Input: part model. Units: mm. Frame: model coordinates. A direction names the side the tool comes from. Give positions to 0.01 mm unless a question says otherwise; leave off trailing zeros. Loops run counter-clockwise (first coordinate to the right, second up) from the corner with the lowest first, then second, coordinate; pieces in that order, holes last. Notation, with made-up numbers: (27, 54.5) - (36, 54.5) arc R19 ccw to (36, 59.5) - close; hole circle Ø10 at (-18, 57). An arc over 180 degrees is marked (long way). Answer as a JSON object with one key per item and string values. Group by question number.
(1) Material intervals for L1, parallel to Y at x = 46, z = 3.5; L2, parallel to Z at x = -50.5, y = 17.25; L3, parallel to Z at x = 42.5, y = 9.75, sorted ascending.
(2) Section query B-B (x = -17). Return loops of the section in (y, z) (3 decimals), plus the area to 3 significant figures.
(3) Mould query, pull axis X, two halves, no side actions, for faces 1 (the cylindrical face through (-0.867, 10.383, -16.587)), 2 (the cylindrical face through (48.4, 25.15, -16.61)), 3 (the flat face through (-1, 0, 0)). Classes: +X half, -X half, draft (parallel to the pull), parting line (faces both ways), or undercut.
(4) Section query A-A (x = 0). Return loops of the section in (y, z), plus the area to 4 significant figures.
(5) Section query C-C (x = 25). Return loops of the section in (y, z), plus the area to 3 significant figures.
(6) Access query for faces 4 (the cylindrical face through (11.195, 0.751, 16.759)), 5 (the cylindrical face through (-55.207, 0.773, -4.883)). Directions: +Z, -Z, +X, -X, +Y, -Y. A direction counts if a zero-diameter tool reaches every point of the face in a straight line with its end or side. Return the directions, or none.
(7) Pin query (flat end, axial travel): P1, Ø1.3, axis at x = -11.41, z = 5.36, coming from the -Y side; P2, Ø3, axis at y = 2.5, z = -1.5, coming from the -X side; P3, Ø0.5, axis at x = 9.5, y = 1, coming from the +Z side; P4, Ø7, axis at x = -53.075, z = 5.5, coming from the +Y side. Return the tip coordinate at first contact, or that it passes through.
```python
from build123d import *

# Parameters (mm, degrees)
SKETCH1_W               = 114.3
SKETCH1_H               = 34.72
BOSS_EXTRUDE1_DEPTH     = 1.524
SKETCH2_R               = 2.184
SKETCH2_W               = 8.15
SKETCH2_H               = 6.35
CUT_EXTRUDE1_DEPTH      = 1.524
SKETCH3_R               = 4
CUT_EXTRUDE2_DEPTH      = 50
SKETCH4_R               = 1.09
CUT_EXTRUDE3_DEPTH      = 50
CIRPATTERN1_COUNT       = 4
MIRROR2_COPY_1_SKETCH_R = 1.09
MIRROR2_COPY_1_DEPTH    = 50
MIRROR2_COPY_2_SKETCH_R = 1.09
MIRROR2_COPY_2_DEPTH    = 50
MIRROR2_COPY_3_SKETCH_R = 1.09
MIRROR2_COPY_3_DEPTH    = 50
SKETCH7_R               = 4
CUT_EXTRUDE4_DEPTH      = 100
SKETCH8_R               = 1.09
CUT_EXTRUDE5_DEPTH      = 100
CIRPATTERN2_COUNT       = 4
MIRROR3_COPY_1_SKETCH_R = 1.09
MIRROR3_COPY_1_DEPTH    = 50
MIRROR3_COPY_2_SKETCH_R = 1.09
MIRROR3_COPY_2_DEPTH    = 50
MIRROR3_COPY_3_SKETCH_R = 1.09
MIRROR3_COPY_3_DEPTH    = 50
MIRROR3_COPY_4_SKETCH_R = 4
MIRROR3_COPY_4_DEPTH    = 50
MIRROR3_COPY_5_SKETCH_R = 1.09
MIRROR3_COPY_5_DEPTH    = 50
MIRROR3_COPY_6_SKETCH_R = 1.09
MIRROR3_COPY_6_DEPTH    = 50
MIRROR3_COPY_7_SKETCH_R = 1.09
MIRROR3_COPY_7_DEPTH    = 50
MIRROR3_COPY_8_SKETCH_R = 1.09
MIRROR3_COPY_8_DEPTH    = 50
SKETCH9_W               = 7.9375
SKETCH9_H               = 1.524
BOSS_EXTRUDE2_DEPTH     = 24.2
SKETCH10_W              = 98
SKETCH10_H              = 1.524
SKETCH10_W_2            = 18.075
BOSS_EXTRUDE3_DEPTH     = 24.2
SKETCH11_R              = 2.1844
CUT_EXTRUDE6_DEPTH      = 24.2
SKETCH12_R              = 2.1844
CUT_EXTRUDE8_DEPTH      = 24.2
FILLET1_R               = 1
SKETCH13_R              = 1.5875
CUT_EXTRUDE9_DEPTH      = 24.2
FILLET2_R               = 2
SKETCH14_R              = 4
CUT_EXTRUDE10_DEPTH     = 24.2
SKETCH15_R              = 1.09
CUT_EXTRUDE11_DEPTH     = 24.2
CIRPATTERN3_COUNT       = 4


with BuildPart() as part:
    # Sketch1 → Boss-Extrude1 (new body)
    with BuildSketch(Plane(origin=(0, 0, 0), x_dir=(1, 0, 0), z_dir=(0, 1, 0))):
        Rectangle(SKETCH1_W, SKETCH1_H)
    extrude(amount=BOSS_EXTRUDE1_DEPTH)

    # Sketch2 → Cut-Extrude1 (cut)
    with BuildSketch(Plane(origin=(0, 1.524, 0), x_dir=(1, 0, 0), z_dir=(0, 1, 0))):
        with Locations(Location((-53.075, 4.41, 0), (0, 0, 270))):
            Circle(SKETCH2_R)
        with Locations(Location((-53.075, -5.5, 0), (0, 0, 270))):
            Circle(SKETCH2_R)
        with Locations((-53.075, 14.185)):
            Rectangle(SKETCH2_W, SKETCH2_H)
        Polygon((-57.15, -13.36), (-49.2125, -13.36), (-49.2125, -9.16), (-47.625, -9.16), (-47.625, -13.36), (-47.625, -17.36), (-57.15, -17.36), align=None)
        Polygon((-10.625, -13.36), (-10.625, -9.16), (-9.0375, -9.16), (-9.0375, -13.36), (0, -13.36), (0, -17.36), (-10.625, -17.36), align=None)
    cut_extrude1 = extrude(amount=-CUT_EXTRUDE1_DEPTH, mode=Mode.SUBTRACT)

    # Mirror1: Cut-Extrude1 across plane
    add(cut_extrude1.mirror(Plane(origin=(0, 0, 0), x_dir=(0, 0, 1), z_dir=(1, 0, 0))), mode=Mode.SUBTRACT)

    # Sketch3 → Cut-Extrude2 (cut, symmetric)
    with BuildSketch(Plane(origin=(0, 1.524, 0), x_dir=(1, 0, 0), z_dir=(0, 1, 0))):
        with Locations(Location((-36.9062, -5.36, 0), (0, 0, 90))):
            Circle(SKETCH3_R)
    cut_extrude2 = extrude(amount=CUT_EXTRUDE2_DEPTH, both=True, mode=Mode.SUBTRACT)

    # Sketch4 → Cut-Extrude3 (cut, symmetric)
    with BuildSketch(Plane(origin=(0, 1.524, 0), x_dir=(1, 0, 0), z_dir=(0, 1, 0))):
        with Locations(Location((-36.9062, 3.14, 0), (0, 0, 90))):
            Circle(SKETCH4_R)
    cut_extrude3 = extrude(amount=CUT_EXTRUDE3_DEPTH, both=True, mode=Mode.SUBTRACT)

    # CirPattern1: Cut-Extrude3 ×4 about axis
    cirpattern1_axis = Axis((-36.9062, 0, 5.36), (0, 1, 0))
    for i in range(1, CIRPATTERN1_COUNT):
        add(cut_extrude3.rotate(cirpattern1_axis, i * 360 / CIRPATTERN1_COUNT), mode=Mode.SUBTRACT)

    # Mirror2: Cut-Extrude2, Cut-Extrude3 across plane
    add(cut_extrude2.mirror(Plane.ZY.offset(28.4062)), mode=Mode.SUBTRACT)
    add(cut_extrude3.mirror(Plane.ZY.offset(28.4062)), mode=Mode.SUBTRACT)

    # Mirror2 copy 1 sketch → Mirror2 copy 1 (cut, symmetric)
    with BuildSketch(Plane(origin=(-14.5462, 1.524, -31.5462), x_dir=(0, 0, -1), z_dir=(0, 1, 0))):
        with Locations((-36.9062, -3.14)):
            Circle(MIRROR2_COPY_1_SKETCH_R)
    extrude(amount=MIRROR2_COPY_1_DEPTH, both=True, mode=Mode.SUBTRACT)

    # Mirror2 copy 2 sketch → Mirror2 copy 2 (cut, symmetric)
    with BuildSketch(Plane(origin=(17, 1.524, 10.72), x_dir=(1, 0, 0), z_dir=(0, 1, 0))):
        with Locations((-36.9062, -3.14)):
            Circle(MIRROR2_COPY_2_SKETCH_R)
    extrude(amount=MIRROR2_COPY_2_DEPTH, both=True, mode=Mode.SUBTRACT)

    # Mirror2 copy 3 sketch → Mirror2 copy 3 (cut, symmetric)
    with BuildSketch(Plane(origin=(-25.2662, 1.524, 42.2662), x_dir=(0, 0, 1), z_dir=(0, 1, 0))):
        with Locations((-36.9062, -3.14)):
            Circle(MIRROR2_COPY_3_SKETCH_R)
    extrude(amount=MIRROR2_COPY_3_DEPTH, both=True, mode=Mode.SUBTRACT)

    # Sketch7 → Cut-Extrude4 (cut)
    with BuildSketch(Plane(origin=(0, 1.524, 0), x_dir=(1, 0, 0), z_dir=(0, 1, 0))):
        with Locations(Location((0, -5.36, 0), (0, 0, 270))):
            Circle(SKETCH7_R)
    extrude(amount=-CUT_EXTRUDE4_DEPTH, mode=Mode.SUBTRACT)

    # Sketch8 → Cut-Extrude5 (cut)
    with BuildSketch(Plane(origin=(0, 1.524, 0), x_dir=(1, 0, 0), z_dir=(0, 1, 0))):
        with Locations(Location((0, 3.14, 0), (0, 0, 270))):
            Circle(SKETCH8_R)
    cut_extrude5 = extrude(amount=-CUT_EXTRUDE5_DEPTH, mode=Mode.SUBTRACT)

    # CirPattern2: Cut-Extrude5 ×4 about axis, 1 skipped
    cirpattern2_axis = Axis((0, 0, 5.36), (0, 1, 0))
    add([cut_extrude5.rotate(cirpattern2_axis, i * 360 / CIRPATTERN2_COUNT) for i in range(1, CIRPATTERN2_COUNT) if i not in (2,)], mode=Mode.SUBTRACT)

    # Mirror3: Cut-Extrude2, Cut-Extrude3 across plane
    add(cut_extrude2.mirror(Plane(origin=(0, 0, 0), x_dir=(0, 0, 1), z_dir=(1, 0, 0))), mode=Mode.SUBTRACT)
    add(cut_extrude3.mirror(Plane(origin=(0, 0, 0), x_dir=(0, 0, 1), z_dir=(1, 0, 0))), mode=Mode.SUBTRACT)

    # Mirror3 copy 1 sketch → Mirror3 copy 1 (cut, symmetric)
    with BuildSketch(Plane(origin=(42.2662, 1.524, -31.5462), x_dir=(0, 0, -1), z_dir=(0, 1, 0))):
        with Locations((-36.9062, -3.14)):
            Circle(MIRROR3_COPY_1_SKETCH_R)
    extrude(amount=MIRROR3_COPY_1_DEPTH, both=True, mode=Mode.SUBTRACT)

    # Mirror3 copy 2 sketch → Mirror3 copy 2 (cut, symmetric)
    with BuildSketch(Plane(origin=(73.8124, 1.524, 10.72), x_dir=(1, 0, 0), z_dir=(0, 1, 0))):
        with Locations((-36.9062, -3.14)):
            Circle(MIRROR3_COPY_2_SKETCH_R)
    extrude(amount=MIRROR3_COPY_2_DEPTH, both=True, mode=Mode.SUBTRACT)

    # Mirror3 copy 3 sketch → Mirror3 copy 3 (cut, symmetric)
    with BuildSketch(Plane(origin=(31.5462, 1.524, 42.2662), x_dir=(0, 0, 1), z_dir=(0, 1, 0))):
        with Locations((-36.9062, -3.14)):
            Circle(MIRROR3_COPY_3_SKETCH_R)
    extrude(amount=MIRROR3_COPY_3_DEPTH, both=True, mode=Mode.SUBTRACT)

    # Mirror3 copy 4 sketch → Mirror3 copy 4 (cut, symmetric)
    with BuildSketch(Plane(origin=(56.8124, 1.524, 0), x_dir=(1, 0, 0), z_dir=(0, 1, 0))):
        with Locations(Location((-36.9062, -5.36, 0), (0, 0, 90))):
            Circle(MIRROR3_COPY_4_SKETCH_R)
    extrude(amount=MIRROR3_COPY_4_DEPTH, both=True, mode=Mode.SUBTRACT)

    # Mirror3 copy 5 sketch → Mirror3 copy 5 (cut, symmetric)
    with BuildSketch(Plane(origin=(56.8124, 1.524, 0), x_dir=(1, 0, 0), z_dir=(0, 1, 0))):
        with Locations(Location((-36.9062, 3.14, 0), (0, 0, 90))):
            Circle(MIRROR3_COPY_5_SKETCH_R)
    extrude(amount=MIRROR3_COPY_5_DEPTH, both=True, mode=Mode.SUBTRACT)

    # Mirror3 copy 6 sketch → Mirror3 copy 6 (cut, symmetric)
    with BuildSketch(Plane(origin=(14.5462, 1.524, -31.5462), x_dir=(0, 0, -1), z_dir=(0, 1, 0))):
        with Locations(Location((-36.9062, 3.14, 0), (0, 0, 90))):
            Circle(MIRROR3_COPY_6_SKETCH_R)
    extrude(amount=MIRROR3_COPY_6_DEPTH, both=True, mode=Mode.SUBTRACT)

    # Mirror3 copy 7 sketch → Mirror3 copy 7 (cut, symmetric)
    with BuildSketch(Plane(origin=(-17, 1.524, 10.72), x_dir=(-1, 0, 0), z_dir=(0, 1, 0))):
        with Locations(Location((-36.9062, 3.14, 0), (0, 0, 90))):
            Circle(MIRROR3_COPY_7_SKETCH_R)
    extrude(amount=MIRROR3_COPY_7_DEPTH, both=True, mode=Mode.SUBTRACT)

    # Mirror3 copy 8 sketch → Mirror3 copy 8 (cut, symmetric)
    with BuildSketch(Plane(origin=(25.2662, 1.524, 42.2662), x_dir=(0, 0, 1), z_dir=(0, 1, 0))):
        with Locations(Location((-36.9062, 3.14, 0), (0, 0, 90))):
            Circle(MIRROR3_COPY_8_SKETCH_R)
    extrude(amount=MIRROR3_COPY_8_DEPTH, both=True, mode=Mode.SUBTRACT)

    # Sketch9 → Boss-Extrude2 (add)
    with BuildSketch(Plane(origin=(0, 1.524, 0), x_dir=(1, 0, 0), z_dir=(0, 1, 0))):
        with Locations((-53.18125, -12.598)):
            Rectangle(SKETCH9_W, SKETCH9_H)
    boss_extrude2 = extrude(amount=BOSS_EXTRUDE2_DEPTH)

    # Mirror4: Boss-Extrude2 across plane
    add(boss_extrude2.mirror(Plane(origin=(0, 0, 0), x_dir=(0, 0, 1), z_dir=(1, 0, 0))))

    # Sketch10 → Boss-Extrude3 (add)
    with BuildSketch(Plane(origin=(0, 1.524, 0), x_dir=(1, 0, 0), z_dir=(0, 1, 0))):
        with Locations((0, 16.598)):
            Rectangle(SKETCH10_W, SKETCH10_H)
        with Locations((0, -12.598)):
            Rectangle(SKETCH10_W_2, SKETCH10_H)
    extrude(amount=BOSS_EXTRUDE3_DEPTH)

    # Sketch11 → Cut-Extrude6 (cut)
    with BuildSketch(Plane.XY.offset(13.36)):
        with Locations((-53.18125, 20.644)):
            Circle(SKETCH11_R)
        with Locations((-53.18125, 10.734)):
            Circle(SKETCH11_R)
    cut_extrude6 = extrude(amount=-CUT_EXTRUDE6_DEPTH, mode=Mode.SUBTRACT)

    # Mirror5: Cut-Extrude6 across plane
    add(cut_extrude6.mirror(Plane(origin=(0, 0, 0), x_dir=(0, 0, 1), z_dir=(1, 0, 0))), mode=Mode.SUBTRACT)

    # Sketch12 → Cut-Extrude8 (cut)
    with BuildSketch(Plane.XY.offset(13.36)):
        with Locations((-5.47125, 20.644)):
            Circle(SKETCH12_R)
        with Locations((-5.47125, 10.734)):
            Circle(SKETCH12_R)
        with Locations((5.47125, 10.734)):
            Circle(SKETCH12_R)
        with Locations((5.47125, 20.644)):
            Circle(SKETCH12_R)
    extrude(amount=-CUT_EXTRUDE8_DEPTH, mode=Mode.SUBTRACT)

    # Fillet1
    fillet1_edges = [part.edges().sort_by_distance(p)[0] for p in [
        (53.18125, 0, 13.36),
        (-53.18125, 1.524, 11.836),
        (53.18125, 1.524, 11.836),
        (-57.15, 0.762, -11.01),
        (0, 1.524, -15.836),
        (0, 1.524, 11.836),
        (-53.18125, 0, 13.36),
        (0, 0, 13.36),
        (0, 0, -17.36),
        (57.15, 0.762, -11.01),
    ]]
    fillet(fillet1_edges, radius=FILLET1_R)

    # Sketch13 → Cut-Extrude9 (cut)
    with BuildSketch(Plane.XY.offset(-15.836)):
        with Locations((36.8628, 14.2875)):
            Circle(SKETCH13_R)
        with Locations((17, 14.2875)):
            Circle(SKETCH13_R)
    cut_extrude9 = extrude(amount=-CUT_EXTRUDE9_DEPTH, mode=Mode.SUBTRACT)

    # Mirror6: Cut-Extrude9 across plane
    add(cut_extrude9.mirror(Plane(origin=(0, 0, 0), x_dir=(0, 0, 1), z_dir=(1, 0, 0))), mode=Mode.SUBTRACT)

    # Fillet2
    fillet2_edges = [part.edges().sort_by_distance(p)[0] for p in [
        (47.625, 0.762, 17.36),
        (10.625, 0.762, 17.36),
        (-57.15, 25.724, 12.598),
        (57.15, 25.724, 12.598),
        (-49, 25.724, -16.598),
        (49, 25.724, -16.598),
        (-47.625, 0.762, 17.36),
        (-10.625, 0.762, 17.36),
    ]]
    fillet(fillet2_edges, radius=FILLET2_R)

    # Sketch14 → Cut-Extrude10 (cut)
    with BuildSketch(Plane.XY.offset(-15.836)):
        with Locations((0, 14.2875)):
            Circle(SKETCH14_R)
    extrude(amount=-CUT_EXTRUDE10_DEPTH, mode=Mode.SUBTRACT)

    # Sketch15 → Cut-Extrude11 (cut)
    with BuildSketch(Plane.XY.offset(-15.836)):
        with Locations((0, 5.7875)):
            Circle(SKETCH15_R)
    cut_extrude11 = extrude(amount=-CUT_EXTRUDE11_DEPTH, mode=Mode.SUBTRACT)

    # CirPattern3: Cut-Extrude11 ×4 about axis, 1 skipped
    cirpattern3_axis = Axis((0, 14.2875, 0), (0, 0, 1))
    add([cut_extrude11.rotate(cirpattern3_axis, i * 360 / CIRPATTERN3_COUNT) for i in range(1, CIRPATTERN3_COUNT) if i not in (2,)], mode=Mode.SUBTRACT)


solid = part.part
```
Recorded:
{
 "1": {"L1": "y = 0 to 1.52", "L2": "z = 11.84 to 13.36", "L3": "z = -17.36 to -15.84"},
 "2": {"outline": "(0, -16.36) arc R1 ccw to (1, -17.36) - (12.7, -17.36) - (12.7, -15.836) - (2.524, -15.836) arc R1 cw to (1.524, -14.836) - (1.524, 2.612) - (0, 2.612) - close; (0, 8.108) - (1.524, 8.108) - (1.524, 17.36) - (0, 17.36) - close; (15.875, -17.36) - (25.724, -17.36) - (25.724, -15.836) - (15.875, -15.836) - close", "area": "76.6 mm^2"},
 "3": {"face 1": "undercut", "face 2": "+X half", "face 3": "draft"},
 "4": {"outline": "(0, -16.36) arc R1 ccw to (1, -17.36) - (4.7, -17.36) - (4.7, -15.84) - (2.52, -15.84) arc R1 cw to (1.52, -14.84) - (1.52, -4.23) - (0, -4.23) - close; (0, -2.05) - (1.52, -2.05) - (1.52, 1.36) - (0, 1.36) - close; (0, 9.36) - (1.52, 9.36) - (1.52, 10.84) arc R1 cw to (2.52, 11.84) - (25.72, 11.84) - (25.72, 13.36) - (1, 13.36) arc R1 ccw to (0, 12.36) - close; (6.88, -17.36) - (10.29, -17.36) - (10.29, -15.84) - (6.88, -15.84) - close; (18.29, -17.36) - (25.72, -17.36) - (25.72, -15.84) - (18.29, -15.84) - close", "area": "89.55 mm^2"},
 "5": {"outline": "(0, -16.36) arc R1 ccw to (1, -17.36) - (25.72, -17.36) - (25.72, -15.84) - (2.52, -15.84) arc R1 cw to (1.52, -14.84) - (1.52, 17.36) - (0, 17.36) - close", "area": "89.8 mm^2"},
 "6": {"face 4": "+Z, +Y, -Y", "face 5": "+Y, -Y"},
 "7": {"P1": "passes through", "P2": "stops at x = -57.15", "P3": "stops at z = 9.16", "P4": "stops at y = 1.52"}
}
